Source: CAD feature listing. Evaluate the final solid. Frame: model axes, mm. Face numbers are marked on the shaded views. A direction names the side the tool comes from. Give positions to 0.01 mm unless a question says otherwise; leave off trailing zeros. Order: outer loops, then holes, each group sorted by start corner. A loop starts at its lowest first (then second) coordinate and runs counter-clockwise, first axis right, second up. Notation, with made-up numbers: M -18.75,-22 L 35.25,-22 A24 ccw 35.25,-1 Z; hole C -24.75,-2 d10. An arc over 180 degrees is marked long. Use CSV: the item, a comma, the result in double quotes. Start each with the question number.
Item 1: Section query D-D on x = -78. Return loops of the section in (y, z), and give its area (3 significant figures).
Item 2: Pull-direction query (X, two-part tool) for the marked faces 1, 2 and 3; classes: +X half, -X half, draft (parallel to the pull), parting line (faces both ways), or undercut.
Item 3: Access query for the marked faces 4, 5 and 6. Directions: +Z, -Z, +X, -X, +Y, -Y. A direction counts if a zero-diameter tool reaches every point of the face in a straight line with its end or side. Return the directions, or none.
Item 4: Ray query, probe 1 along Z at (x, y) = (-72, -6); probe 2 along Y at (x, z) = (-21.5, 4); probe 3 along Y at (x, z) = (0, 8). Return the intervals inside material, ascending. Write a range as from..to.
Item 5: Section query C-C on z = 18. Return loops of the section in (x, y), and give its area (3 significant figures).
Item 6: Section query A-A on x = 0. Return loops of the section in (y, z), and give its area (3 significant figures).
Item 7: Section query B-B on y = 0. Return loops of the section in (x, z), and give its area (3 significant figures).
Item 8: First-contact query: pin 1 (1 mm diameter, centred on x = -26.5, z = 23, fed in from +Y); pin 2 (11.5 mm diameter, centred on x = -41.5, z = 28.5, fed in from -Y); pin 3 (6 mm diameter, centred on x = -100.5, z = 9, fed in from -Y). Flat tips, straight axial feed; report the tip coordinate or a pass-through.
from build123d import *

# Parameters (mm, degrees)
SKETCH1_R                = 20
SKETCH1_R_2              = 14.505051228
BOSS_EXTRUDE1_DEPTH      = 4
BOSS_EXTRUDE2_DEPTH      = 15.075
SKETCH3_R                = 5.05
CUT_EXTRUDE1_DEPTH       = 51.075
SKETCH4_R                = 2.5
BOSS_EXTRUDE3_DEPTH      = 32
BOSS_EXTRUDE3_DEPTH_BACK = 2


with BuildPart() as part:
    # Sketch1 → Boss-Extrude1 (new body)
    with BuildSketch(Plane.XY):
        Circle(SKETCH1_R)
        with BuildLine():
            Line((-99.203276416, -14.505051228), (-13.76965827, -14.505051228))
            ThreePointArc((-13.76965827, -14.505051228), (-20, 0), (-13.76965827, 14.505051228))
            Line((-13.76965827, 14.505051228), (-99.203276416, 14.505051228))
            ThreePointArc((-99.203276416, 14.505051228), (-88.946656331, 10.256620085), (-84.698225188, 0))
            ThreePointArc((-84.698225188, 0), (-88.946656331, -10.256620085), (-99.203276416, -14.505051228))
        make_face()
        with Locations((-99.203276416, 0)):
            Circle(SKETCH1_R_2)
    extrude(amount=BOSS_EXTRUDE1_DEPTH)

    # Sketch2 → Boss-Extrude2 (add)
    with BuildSketch(Plane.XY.offset(4)):
        with BuildLine():
            Line((-13.76965827, 14.505051228), (-81.604060492, 14.505051228))
            ThreePointArc((-81.604060492, 14.505051228), (-67.970381175, 0), (-81.604060492, -14.505051228))
            Line((-81.604060492, -14.505051228), (-13.76965827, -14.505051228))
            ThreePointArc((-13.76965827, -14.505051228), (20, 0), (-13.76965827, 14.505051228))
        make_face()
    extrude(amount=BOSS_EXTRUDE2_DEPTH)

    # Mirror1: part across plane


with BuildPart() as part_1:
    add(part.part)
    add(part.part.mirror(Plane.XY.offset(19.075)))

    # Sketch3 → Cut-Extrude1 (cut)
    with BuildSketch(Plane(origin=(0, 0, 0), x_dir=(-1, 0, 0), z_dir=(0, 0, -1))):
        Circle(SKETCH3_R)
    extrude(amount=-CUT_EXTRUDE1_DEPTH, mode=Mode.SUBTRACT)

    # Sketch4 → Boss-Extrude3 (add, two sides)
    with BuildSketch(Plane(origin=(0, 0, 34.15), x_dir=(-1, 0, 0), z_dir=(0, 0, -1))) as boss_extrude3_sk:
        with Locations((99.203276416, 7.252525614)):
            Circle(SKETCH4_R)
        with Locations((99.203276416, -7.252525614)):
            Circle(SKETCH4_R)
    extrude(amount=BOSS_EXTRUDE3_DEPTH)
    extrude(boss_extrude3_sk.sketch, amount=-BOSS_EXTRUDE3_DEPTH_BACK)


solid = part_1.part
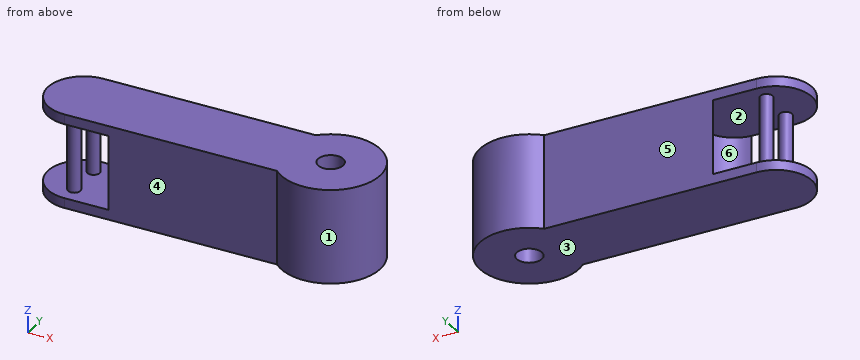
Verdict:
1,outline,"M -14.51,0 L 14.51,0 L 14.51,38.15 L -14.51,38.15 Z; hole M -13.82,4 L 13.82,4 L 13.82,34.15 L -13.82,34.15 Z"
1,area,"274 mm2"
2,face 1,"parting line"
2,face 2,"undercut"
2,face 3,"draft"
3,face 4,"+Z, -Z, -X, -Y"
3,face 5,"+Z, -Z, -X, +Y"
3,face 6,"none"
4,probe 1,"0..4, 34.15..38.15"
4,probe 2,"-14.51..14.51"
4,probe 3,"-20..-5.05, 5.05..20"
5,outline,"C -99.2,-7.25 d5; C -99.2,7.25 d5; M -81.6,-14.51 L -13.77,-14.51 A20 ccw long -13.77,14.51 L -81.6,14.51 A14.53 cw Z; hole C 0,0 d10.1"
5,area,"2,750 mm2"
6,outline,"M -20,0 L -5.05,0 L -5.05,38.15 L -20,38.15 Z; M 5.05,0 L 20,0 L 20,38.15 L 5.05,38.15 Z"
6,area,"1,140 mm2"
7,outline,"M -113.71,0 L -5.05,0 L -5.05,38.15 L -113.71,38.15 L -113.71,34.15 L -67.97,34.15 L -67.97,4 L -113.71,4 Z; M 5.05,0 L 20,0 L 20,38.15 L 5.05,38.15 Z"
7,area,"3,340 mm2"
8,pin 1,"y = 14.51"
8,pin 2,"y = -14.51"
8,pin 3,"y = -9.75"
